Model file for the job. Use its own axes, mm. A direction names the side the tool comes from. Round coordinates to 2 decimals unless told otherwise and drop trailing zeros. Write each loop counter-clockwise with the first axis right and the second up, starting at its lowest first coordinate (ties: lowest second). Pieces come first, ordered by that corner, then holes. Notation, with made-up numbers: (9.5, 52) - (25.5, 52) arc R3 ccw to (25.5, 56) - close; hole circle Ø11 at (66, 70.5). An arc over 180 degrees is marked (long way). Answer as a JSON object with one key per item and string values. Group by question number.
from build123d import *

# Parameters (mm, degrees)
F0_W     = 4
F0_H     = 50
F1_DEPTH = 25
F2_W     = 50
F2_H     = 4
F3_DEPTH = 25
F4_R     = 15
F5_DEPTH = 25


with BuildPart() as f1:
    # F0 (on Front) → F1 (new body, symmetric)
    with BuildSketch(Plane.XZ):
        with Locations((0, -25)):
            Rectangle(F0_W, F0_H)
    extrude(amount=F1_DEPTH, both=True)

    # F2 (on Front) → F3 (join, symmetric)
    with BuildSketch(Plane.XZ):
        with Locations((0, 2)):
            Rectangle(F2_W, F2_H)
    extrude(amount=F3_DEPTH, both=True)

    # F4 (on Front) → F5 (join, symmetric)
    with BuildSketch(Plane.XZ):
        with Locations((0, -64.434606)):
            Circle(F4_R)
    extrude(amount=F5_DEPTH, both=True)


solid = f1.part
(1) Slice it at B-B (y = 6.5). Write the cut outline in (x, z).
(2) Pull direction Z, two halves, no side cores. Call faces 1 (the flat face through (25, 0, 2)), 2 (the flat face through (0, 0, 4)), 3 (the flat face through (13, 0, 0)): pulls with the +Z half, pulls with the -Z half, needs draft (parallel to the pull), parting line crosses it, or undercut.
(3) Slice it at A-A (x = -12). Write the cut outline in (y, z).
(4) 3-axis set-ups, long thin cutter, end or side, ignore diameter. For faces 4 (the flat face through (-14, 0, 0)), 5 (the flat face through (1.7, 25, -46.8)), 6 (the flat face through (2, 0, -25)): which of +Z, -Z, +X, -X, +Y, -Y reach the whole face in a straight line?
(5) Flat gauge pins, fed straight in: pin 1 (2 mm diameter, centred on y = 4.5, z = -61.5, fed in from -X); pin 2 (11.5 mm diameter, centred on x = -13, y = 12, fed in from -Z); pin 3 (7 mm diameter, centred on x = 19, y = -11.5, fed in from -Z). Where does each tip first touch, or does it go through?
(6) Slice it at C-C (x = 19). Write the cut outline in (y, z).
(7) Drill centre lines: line 1 (Z direction, x = -22, y = 13.5); line 2 (Z direction, x = 9, y = 11); line 3 (X direction, y = -4, z = -6). Where is each one in solid material? Low to high. Write a range as from..to.
(8) Slice it at D-D (z = -18). Write the cut outline in (x, y).
Answer:
{
 "1": {"outline": "(-25, 0) - (-2, 0) - (-2, -49.57) arc R15 ccw (long way) to (2, -49.57) - (2, 0) - (25, 0) - (25, 4) - (-25, 4) - close"},
 "2": {"face 1": "needs draft", "face 2": "pulls with the +Z half", "face 3": "undercut"},
 "3": {"outline": "(-25, -73.43) - (25, -73.43) - (25, -55.43) - (-25, -55.43) - close; (-25, 0) - (25, 0) - (25, 4) - (-25, 4) - close"},
 "4": {"face 4": "-X, +Y, -Y", "face 5": "+Z, -Z, +X, -X, +Y", "face 6": "+X, +Y, -Y"},
 "5": {"pin 1": "x = -14.87", "pin 2": "z = -77.57", "pin 3": "z = 0"},
 "6": {"outline": "(-25, 0) - (25, 0) - (25, 4) - (-25, 4) - close"},
 "7": {"line 1": "0..4", "line 2": "-76.43..-52.43, 0..4", "line 3": "-2..2"},
 "8": {"outline": "(-2, -25) - (2, -25) - (2, 25) - (-2, 25) - close"}
}
